from build123d import *

# Parameters (mm, degrees)
F0_W     = 971.55
F0_H     = 177.8
F1_DEPTH = 3.175
F2_R     = 9.525
F3_DEPTH = 133.35
F4_DEPTH = 38.1


with BuildPart() as f1:
    # F0 (on Top) → F1 (new body)
    with BuildSketch(Plane.XY):
        with Locations((485.775, -88.9)):
            Rectangle(F0_W, F0_H)
    extrude(amount=F1_DEPTH)

    # F2 (on face) → F3 (join)
    with BuildSketch(Plane.XY.offset(3.175)):
        with Locations((43.688, -88.9)):
            Circle(F2_R)
        with BuildLine():
            ThreePointArc((313.563, -88.9), (304.038, -79.375), (294.513, -88.9))
            ThreePointArc((294.513, -88.9), (304.038, -98.425), (313.563, -88.9))
        make_face()
        with Locations((355.6, -88.9)):
            Circle(F2_R)
        with BuildLine():
            ThreePointArc((625.475, -88.9), (615.95, -79.375), (606.425, -88.9))
            ThreePointArc((606.425, -88.9), (615.95, -98.425), (625.475, -88.9))
        make_face()
        with Locations((666.75, -88.9)):
            Circle(F2_R)
        with BuildLine():
            ThreePointArc((917.575, -88.9), (927.1, -98.425), (936.625, -88.9))
            ThreePointArc((936.625, -88.9), (927.1, -79.375), (917.575, -88.9))
        make_face()
    extrude(amount=F3_DEPTH)

    # F4 (add): faces of the model
    f4_faces = [f1.faces().sort_by_distance(p)[0] for p in [
        (355.6, -88.9, 136.525),
        (615.95, -88.9, 136.525),
    ]]
    extrude(f4_faces, amount=F4_DEPTH)


solid = f1.part
Model file for the job. Use its own axes, mm. A direction names the side the tool comes from. Give positions to 0.01 mm unless a question says otherwise; leave off trailing zeros. Loops run counter-clockwise (first coordinate to the right, second up) from the corner with the lowest first, then second, coordinate; pieces in that order, holes last. Notation, with made-up numbers: (84, 78.25) - (102, 78.25) arc R30 cw to (102, 117.25) - close; hole circle Ø4 at (-40, -39). An arc over 180 degrees is marked (long way). Use one line per item in the form item = value.
(1) Drop flat-ended pins along their axis: P1, Ø5.5, axis at x = 45, y = -85, coming from the +Z side (3 decimals); P2, Ø5, axis at y = -84.5, z = 59.5, coming from the +X side; P3, Ø10, axis at y = -84, z = 132.5, coming from the +X side (3 decimals). Give the stop position or say it passes through.
Determined:
P1 = 136.525
P2 = 936.43
P3 = 936.625
(2) Pull direction X, two halves, no side cores. Call faces 4 (the face through (355, -89, 174.625)), 5 (the face through (364.685, -86.039, 87.7)): pulls with the +X half, pulls with the -X half, needs draft (parallel to the pull), parting line crosses it, or undercut.
Determined:
face_4 = needs draft
face_5 = undercut
(3) Drill centre lines: L1, parallel to X at y = -94, z = 48.5; L2, parallel to Z at x = 41.5, y = -30.5 (3 decimals); L3, parallel to Y at x = 675, z = 130. Where is each one in solid material? Low to high.
Determined:
L1 = 35.64 to 51.73, 295.99 to 312.08, 347.56 to 363.64, 607.91 to 623.99, 658.71 to 674.79, 919.06 to 935.14
L2 = 0 to 3.175
L3 = -93.66 to -84.14
(4) Cut at D-D (z = 149). Give the cut face in (x, y) (3 decimals).
Determined:
outline = circle Ø19.05 at (355.6, -88.9); circle Ø19.05 at (615.95, -88.9)
(5) Cut at A-A (z = 16). Give the cut face in (x, y) (3 decimals).
Determined:
outline = circle Ø19.05 at (43.688, -88.9); circle Ø19.05 at (304.038, -88.9); circle Ø19.05 at (355.6, -88.9); circle Ø19.05 at (615.95, -88.9); circle Ø19.05 at (666.75, -88.9); circle Ø19.05 at (927.1, -88.9)
(6) Cut at B-B (x = 927.1). Give the cut face in (y, z) (3 decimals).
Determined:
outline = (-177.8, 0) - (0, 0) - (0, 3.175) - (-79.375, 3.175) - (-79.375, 136.525) - (-98.425, 136.525) - (-98.425, 3.175) - (-177.8, 3.175) - close
(7) 3-axis set-ups, long thin cutter, end or side, ignore diameter. For faces 1 (the face through (42.448, -79.456, 68.917)), 2 (the face through (927, -89, 136.525)), 3 (the face through (304, -89, 136.525)): which of +Z, -Z, +X, -X, +Y, -Y reach the whole face in a straight line?
Determined:
face_1 = +Z
face_2 = +Z, +X, +Y, -Y
face_3 = +Z, -X, +Y, -Y
(8) Cut at C-C (y = -88.9). Give the cut face in (x, z) (3 decimals).
Determined:
outline = (0, 0) - (971.55, 0) - (971.55, 3.175) - (936.625, 3.175) - (936.625, 136.525) - (917.575, 136.525) - (917.575, 3.175) - (676.275, 3.175) - (676.275, 136.525) - (657.225, 136.525) - (657.225, 3.175) - (625.475, 3.175) - (625.475, 174.625) - (606.425, 174.625) - (606.425, 3.175) - (365.125, 3.175) - (365.125, 174.625) - (346.075, 174.625) - (346.075, 3.175) - (313.563, 3.175) - (313.563, 136.525) - (294.513, 136.525) - (294.513, 3.175) - (53.213, 3.175) - (53.213, 136.525) - (34.163, 136.525) - (34.163, 3.175) - (0, 3.175) - close
